Verification items for the finished model (mm, model axes). A direction names the side the tool comes from. Coordinates: 2 decimals unless noted, no trailing zeros. Write each loop counter-clockwise with the first axis right and the second up, starting at its lowest first coordinate (ties: lowest second). Pieces come first, ordered by that corner, then holes. Notation, with made-up numbers: (22, 60.5) -> (65, 60.5) arc R14 ccw to (65, 76.5) -> close; hole circle Ø10 at (-30, -14). An arc over 180 degrees is marked (long way). Answer in a Markdown table with one row per item.
```python
from build123d import *

# Parameters (mm, degrees)
F1_DEPTH    = 25.4
F2_R        = 15.24
F3_T1_DEPTH = 36.0903109365
F4_W        = 3.5194646057
F4_H        = 9.0122472823
F4_W_2      = 2.8517952656
F4_W_3      = 4.2412726252
F5_DEPTH    = 25.4


# Not quite as in the source:
# - a fillet or chamfer that OpenCascade refuses, or shapes differently, is made with other operations: its cross-section is extruded or revolved along the edge and cut away or added


with BuildPart() as f1:
    # F0 (on Top) → F1 (new body)
    with BuildSketch(Plane.XY):
        with BuildLine():
            ThreePointArc((-13.0763784004, -10.4391818642), (0, 16.73225), (13.0763784004, -10.4391818642))
            Line((13.0763784004, -10.4391818642), (13.0763784004, -15.0102275297))
            ThreePointArc((13.0763784004, -15.0102275297), (19.2516474294, -5.0668208785), (18.7713860197, 6.6282478426))
            Line((18.7713860197, 6.6282478426), (62.8066707781, -6.8086651928))
            ThreePointArc((62.8066707781, -6.8086651928), (65.147620689, -13.3496506564), (58.2099580532, -13.7148553544))
            Line((58.2099580532, -13.7148553544), (55.7661979944, -15.7418387719))
            ThreePointArc((55.7661979944, -15.7418387719), (67.7906892269, -15.1088589169), (63.7333095074, -3.7718962412))
            Line((63.7333095074, -3.7718962412), (16.9015827692, 10.5183222263))
            ThreePointArc((16.9015827692, 10.5183222263), (-12.9067718767, 15.1563136113), (-13.0763784004, -15.0102275297))
            Line((-13.0763784004, -15.0102275297), (-13.0763784004, -10.4391818642))
        make_face()
    extrude(amount=F1_DEPTH)

    # F2
    f2_edges = [f1.edges().sort_by_distance(p)[0] for p in [
        (16.901583, 10.518322, 12.7),
        (18.771386, 6.628248, 12.7),
    ]]
    fillet(f2_edges, radius=F2_R)

    # F3: chamfer of 2.54 on 1 edges, made by hand

    # F3_s2 → F3_t1 (cut)
    with BuildSketch(Plane.XY.offset(-5.3451554683)):
        with BuildLine():
            Line((59.4681740413, -14.7511998168), (56.6296179231, -15.0256727671))
            Line((56.6296179231, -15.0256727671), (58.2099580532, -13.7148553544))
            ThreePointArc((58.2099580532, -13.7148553544), (58.8184317915, -14.3160957873), (59.4681740413, -14.7511998168))
        make_face()
    extrude(amount=F3_T1_DEPTH, mode=Mode.SUBTRACT)

    # F4 (on face) → F5 (cut)
    with BuildSketch(Plane(origin=(1.9640154801, -20.3115394411, 0), x_dir=(-0.9953576095, -0.0962456715, 0), z_dir=(-0.0962456715, 0.9953576095, 0))):
        with Locations((-59.5320927234, 8.1938763589)):
            Rectangle(F4_W, F4_H)
        with Locations((-59.5320927234, 17.2061236411)):
            Rectangle(F4_W, F4_H)
        with Locations((-56.3464627878, 17.2061236411)):
            Rectangle(F4_W_2, F4_H)
        with Locations((-56.3464627878, 8.1938763589)):
            Rectangle(F4_W_2, F4_H)
        with Locations((-52.7999288424, 8.1938763589)):
            Rectangle(F4_W_3, F4_H)
        with Locations((-52.7999288424, 17.2061236411)):
            Rectangle(F4_W_3, F4_H)
    extrude(amount=-F5_DEPTH, mode=Mode.SUBTRACT)


solid = f1.part
```
1. Mould release check, pull along Z, two halves, no side actions. Record for faces 4 (the flat face through (58.069, -14.887, 23.53)), 5 (the flat face through (63.183, -16.605, 12.826)), 6 (the flat face through (21, 2, 0)), 7 (the flat face through (60, -17, 21.712)): released by +Z, released by -Z, zero draft, split by the parting line, or undercut.
Geometry says:
| item | result |
|---|---|
| face 4 | zero draft |
| face 5 | undercut |
| face 6 | released by -Z |
| face 7 | undercut |
2. Section check A-A, the plane y = 0. Record the boundary of the cut face in (x, z), plus the area to 3 significant figures.
Geometry says:
| item | result |
|---|---|
| outline | (-19.91, 0) -> (-16.73, 0) -> (-16.73, 25.4) -> (-19.91, 25.4) -> close; (16.73, 0) -> (25.35, 0) -> (25.35, 25.4) -> (16.73, 25.4) -> close; (40.49, 0) -> (51.37, 0) -> (51.37, 25.4) -> (40.49, 25.4) -> close |
| area | 576 mm^2 |
3. Section check D-D, the plane y = -12. Record the boundary of the cut face in (x, z).
Geometry says:
| item | result |
|---|---|
| outline | (-15.88, 0) -> (-13.08, 0) -> (-13.08, 25.4) -> (-15.88, 25.4) -> close; (13.08, 0) -> (15.88, 0) -> (15.88, 25.4) -> (13.08, 25.4) -> close; (65.74, 0) -> (68.97, 0) -> (68.97, 25.4) -> (65.74, 25.4) -> close |
4. Thickness scan on line 1 (X direction, y = -9, z = 15.25); line 2 (X direction, y = -11.5, z = 4.75); line 3 (Y direction, x = -0.5, z = 22.25). Record the ranges inside material, lowest first. Write a range as from..to.
Geometry says:
| item | result |
|---|---|
| line 1 | -17.76..-14.11, 14.11..17.76, 65.41..68.79 |
| line 2 | -16.25..-13.08, 13.08..16.25, 65.84..69.03 |
| line 3 | 16.72..19.9 |
5. Section check C-C, the plane x = 0. Record the boundary of the cut face in (y, z), plus the area to 3 significant figures.
Geometry says:
| item | result |
|---|---|
| outline | (16.73, 0) -> (19.91, 0) -> (19.91, 25.4) -> (16.73, 25.4) -> close |
| area | 80.6 mm^2 |
6. Tool access check on faces 1 (the flat face through (58.069, -14.887, 1.818)), 2 (the cylindrical face through (16.12, -11.68, 12.52)), 3 (the flat face through (21, 2, 25.4)). Record the directions out of +Z, -Z, +X, -X, +Y, -Y that give a thin tool (end or side, any length) a straight path to the whole face; none if there is none.
Geometry says:
| item | result |
|---|---|
| face 1 | +Z, -Z |
| face 2 | +Z, -Z, -Y |
| face 3 | +Z, +X, -X, +Y, -Y |
7. Section check B-B, the plane z = 14.5. Record the boundary of the cut face in (x, y), plus the area to 3 significant figures.
Geometry says:
| item | result |
|---|---|
| outline | (-13.08, -15.01) -> (-13.08, -10.44) arc R16.73 cw (long way) to (13.08, -10.44) -> (13.08, -15.01) arc R19.91 ccw to (18.38, -7.64) arc R15.24 cw to (36.91, 1.09) -> (62.81, -6.81) arc R4.33 cw to (63.03, -15.02) -> (63.34, -18.24) arc R7.51 ccw to (63.73, -3.77) -> (21.52, 9.11) arc R15.24 cw to (14.71, 13.42) arc R19.91 ccw (long way) to start |
| area | 536 mm^2 |
8. Depth check by flat-ended pin: P1, Ø3, axis at y = 13, z = 20.5, coming from the +X side; P2, Ø5, axis at y = -13.5, z = 7.5, coming from the -X side; P3, Ø11.5, axis at x = 61.54, y = -10.95, coming from the -Z side; P4, Ø3, axis at x = 47, y = 4.5, coming from the +Z side. Enter the tip coordinate at first touch or a pass-through.
Geometry says:
| item | result |
|---|---|
| P1 | x = 16.82 |
| P2 | x = -16.59 |
| P3 | z = 0 |
| P4 | through |
